Check sheet for the modelled part. Datum: model origin and axes. Units: mm. A direction names the side the tool comes from. Round coordinates to 2 decimals unless told otherwise and drop trailing zeros. Write each loop counter-clockwise with the first axis right and the second up, starting at its lowest first coordinate (ties: lowest second). Pieces come first, ordered by that corner, then holes.
Item 1: Set-up check for faces 1 (the flat face through (-2, -22.5, 185)), 2 (the flat face through (-5, -2, 177)), 3 (the flat face through (-5.4, 14.12, 180.55)): record each of +Z, -Z, +X, -X, +Y, -Y from which the full face is reachable in a straight line by a thin tool's end or side.
Item 2: Release check for a two-part mould opening along Z. For faces 4 (the flat face through (-6, 0, -226)), 5 (the flat face through (-382, 14, -3)), 6 (the flat face through (-426.5, 0, -3)), 7 (the flat face through (-5, -2, -177)) record: pulls with the +Z half, pulls with the -Z half, needs draft (parallel to the pull), parting line crosses it, or undercut.
Item 3: Material ranges on line 1 along X through (y, z) = (3.5, 25); line 2 along Z through (x, y) = (-17.5, 3.5); line 3 along X through (y, z) = (6, -30), recorded low to high.
Item 4: Section check A-A, the plane x = -180.5. Record the cut outline in (y, z), plus the area to 3 significant figures.
Item 5: Section check B-B, the plane z = -166. Record the cut outline in (x, y).
from build123d import *

# Parameters (mm, degrees)
F0_W     = 853
F0_H     = 452
F0_W_2   = 757
F0_H_2   = 354
F1_DEPTH = 22.5
F2_SIZE2 = 13
F2_SIZE  = 6
F3_SIZE2 = 7
F3_SIZE  = 17


with BuildPart() as f1:
    # F0 (on Front) → F1 (new body, symmetric)
    with BuildSketch(Plane.XZ):
        Rectangle(F0_W, F0_H)
        Rectangle(F0_W_2, F0_H_2, mode=Mode.SUBTRACT)
    extrude(amount=F1_DEPTH, both=True)

    # F2
    f2_edges = [f1.edges().sort_by_distance(p)[0] for p in [
        (0, -22.5, -177),
        (-378.5, -22.5, 0),
        (378.5, -22.5, 0),
        (0, -22.5, 177),
    ]]
    chamfer(f2_edges, length=F2_SIZE, length2=F2_SIZE2)

    # F3
    f3_edges = [f1.edges().sort_by_distance(p)[0] for p in [
        (0, 22.5, -177),
        (-378.5, 22.5, 0),
        (0, 22.5, 177),
        (378.5, 22.5, 0),
    ]]
    chamfer(f3_edges, length=F3_SIZE, length2=F3_SIZE2)


solid = f1.part
Values found:
1. face 1: +Z, -Z, +X, -X, -Y
1. face 2: +Y, -Y
1. face 3: +Y
2. face 4: pulls with the -Z half
2. face 5: undercut
2. face 6: needs draft
2. face 7: undercut
3. line 1: x = -426.5 to -378.5, 378.5 to 426.5
3. line 2: z = -226 to -177, 177 to 226
3. line 3: x = -426.5 to -378.71, 378.71 to 426.5
4. outline: (-22.5, -226) - (22.5, -226) - (22.5, -184) - (5.5, -177) - (-9.5, -177) - (-22.5, -183) - close; (-22.5, 183) - (-9.5, 177) - (5.5, 177) - (22.5, 184) - (22.5, 226) - (-22.5, 226) - close
4. area: 4,210 mm2
5. outline: (-426.5, -22.5) - (-384.5, -22.5) - (-378.5, -9.5) - (-378.5, 5.5) - (-385.5, 22.5) - (-426.5, 22.5) - close; (378.5, -9.5) - (384.5, -22.5) - (426.5, -22.5) - (426.5, 22.5) - (385.5, 22.5) - (378.5, 5.5) - close
